from build123d import *

# Parameters (mm, degrees)
EXTRUDE_1_DEPTH   = 2
HOLE_WIZARD_M81_D = 9
CHAMFER_1_SIZE    = 2


with BuildPart() as part:
    # Эскиз1 → Бобышка-Вытянуть1 (new body)
    with BuildSketch(Plane(origin=(0, 0, 0), x_dir=(1, 0, 0), z_dir=(0, 0, -1))):
        Polygon((0, 0), (0, 80), (80, 80), (80, 40), (40, 40), (40, 0), align=None)
    extrude(amount=EXTRUDE_1_DEPTH)

    # Отверстие с зазором M81 (through all)
    with Locations(Plane(origin=(0, 0, -2), x_dir=(1, 0, 0), z_dir=(0, 0, -1))):
        with Locations((20, 60), (20, 20), (60, 60)):
            Hole(HOLE_WIZARD_M81_D / 2)

    # Фаска1
    chamfer_1_edges = [part.edges().sort_by_distance(p)[0] for p in [
        (0, 0, -1),
        (0, -80, -1),
        (80, -80, -1),
        (80, -40, -1),
        (40, 0, -1),
    ]]
    chamfer(chamfer_1_edges, length=CHAMFER_1_SIZE)


solid = part.part
Verification items for the finished model (mm, model axes). Coordinates: 2 decimals unless noted, no trailing zeros. Loops run counter-clockwise (first coordinate to the right, second up) from the corner with the lowest first, then second, coordinate; pieces in that order, holes last. Notation, with made-up numbers: M -24.5,46.5 L 18.5,46.5 A24 cw 18.5,67.5 Z; hole C 40.5,20 d5. An arc over 180 degrees is marked long. One line per item, written item: value.
1. Material ranges on line 1 along Y through (x, z) = (20, -1); line 2 along X through (y, z) = (-60, -1.45); line 3 along X through (y, z) = (-20, -1.1), recorded low to high. Write a range as from..to.
Answers follow:
line 1: -80..-64.5, -55.5..-24.5, -15.5..0
line 2: 0..15.5, 24.5..55.5, 64.5..80
line 3: 0..15.5, 24.5..40
2. Section check B-B on y = -60. Record the cut outline in (x, z), plus the area to 3 significant figures.
Answers follow:
outline: M 0,-2 L 15.5,-2 L 15.5,0 L 0,0 Z; M 24.5,-2 L 55.5,-2 L 55.5,0 L 24.5,0 Z; M 64.5,-2 L 80,-2 L 80,0 L 64.5,0 Z
area: 124 mm^2
3. Section check C-C on y = -20. Record the cut outline in (x, z).
Answers follow:
outline: M 0,-2 L 15.5,-2 L 15.5,0 L 0,0 Z; M 24.5,-2 L 40,-2 L 40,0 L 24.5,0 Z
4. Mould release check, pull along Y, two halves, no side actions. Record for faces 1 (the flat face through (40, -21, -1)), 2 (the flat face through (59, -40, -1)), 3 (the cylindrical face through (23.32, -23.04, -0.99)), 4 (the cylindrical face through (55.708, -61.352, -0.986)): pulls with the +Y half, pulls with the -Y half, needs draft (parallel to the pull), parting line crosses it, or undercut.
Answers follow:
face 1: needs draft
face 2: pulls with the +Y half
face 3: undercut
face 4: undercut
5. Section check D-D on x = 60. Record the cut outline in (y, z), plus the area to 3 significant figures.
Answers follow:
outline: M -80,-2 L -64.5,-2 L -64.5,0 L -80,0 Z; M -55.5,-2 L -40,-2 L -40,0 L -55.5,0 Z
area: 62.0 mm^2
6. Gauge pin test, flat end, axial feed: P1, Ø1, axis at y = -15.5, z = -1, coming from the +X side. Record the tip position at first contact, or that the pin passes through.
Answers follow:
P1: x = 40
7. Section check A-A on x = 20. Record the cut outline in (y, z).
Answers follow:
outline: M -80,-2 L -64.5,-2 L -64.5,0 L -80,0 Z; M -55.5,-2 L -24.5,-2 L -24.5,0 L -55.5,0 Z; M -15.5,-2 L 0,-2 L 0,0 L -15.5,0 Z
